from build123d import *

# Parameters (mm, degrees)
F1_DEPTH = 19.05
F2_R     = 2.5
F3_DEPTH = 1.9
F4_R     = 1.5
F5_DEPTH = 1.9


with BuildPart() as f1:
    # F0 (on Front) → F1 (new body)
    with BuildSketch(Plane.XZ):
        with BuildLine():
            Line((-18.746637599, 0), (31.253362401, 0))
            Line((31.253362401, 0), (31.253362401, 1.9))
            Line((31.253362401, 1.9), (-18.746637599, 1.9))
            ThreePointArc((-18.746637599, 1.9), (-21.0563364303, 3.4432914191), (-20.514404552, 6.167766953))
            Line((-20.514404552, 6.167766953), (-2.8367350223, 23.8454364826))
            Line((-2.8367350223, 23.8454364826), (-4.1802379066, 25.1889393669))
            Line((-4.1802379066, 25.1889393669), (-21.8579074362, 7.5112698372))
            ThreePointArc((-21.8579074362, 7.5112698372), (-22.8117075421, 2.7161928976), (-18.746637599, 0))
        make_face()
    extrude(amount=F1_DEPTH)

    # F2 (on face) → F3 (cut, through all)
    with BuildSketch(Plane.XY.offset(1.9)):
        with Locations((-0.746637599, -9.525)):
            Circle(F2_R)
        with BuildLine():
            ThreePointArc((24.1869203746, -12.025), (26.6482556642, -9.525), (24.1869203746, -7.025))
            Line((24.1869203746, -7.025), (24.1089835763, -7.025))
            Line((24.1089835763, -7.025), (14.3277980387, -7.025))
            ThreePointArc((14.3277980387, -7.025), (11.8277980387, -9.525), (14.3277980387, -12.025))
            Line((14.3277980387, -12.025), (24.1869203746, -12.025))
        make_face()
        with BuildLine():
            Line((24.1089835763, -7.025), (24.1869203746, -7.025))
            ThreePointArc((24.1869203746, -7.025), (24.1479519755, -7.0246963112), (24.1089835763, -7.025))
        make_face()
    extrude(amount=-F3_DEPTH, mode=Mode.SUBTRACT)

    # F4 (on face) → F5 (cut, through all)
    with BuildSketch(Plane(origin=(-14.6845886367, 0, 14.6845886367), x_dir=(0, -1, 0), z_dir=(-0.7071067812, 0, 0.7071067812))):
        with Locations((14.55, 7.3553952665)):
            Circle(F4_R)
        with Locations((4.5, 7.3553952665)):
            Circle(F4_R)
    extrude(amount=-F5_DEPTH, mode=Mode.SUBTRACT)


solid = f1.part
Design review of the part built by this model. Coordinates are the model's own, in mm. A direction names the side the tool comes from. Round coordinates to 2 decimals unless told otherwise and drop trailing zeros. Order: outer loops, then holes, each group sorted by start corner. A loop starts at its lowest first (then second) coordinate and runs counter-clockwise, first axis right, second up.
1) For L1, parallel to X at y = -10.25, z = 1.25; L2, parallel to X at y = -10, z = 1.25; L3, parallel to Z at x = -18.5, y = -4, list the stretches that pass through material, from the lowest coordinate up.
The answers:
L1: x = -21.82 to -3.14, 1.65 to 11.94, 26.54 to 31.25
L2: x = -21.82 to -3.2, 1.71 to 11.87, 26.6 to 31.25
L3: z = 0 to 1.9, 8.18 to 10.87
2) Consider section C-C (y = -8.75). State the section outline as (x, z) points, plus the area to 3 significant figures.
The answers:
outline: (-21.86, 7.51) arc R4.4 ccw to (-18.75, 0) - (-3.12, 0) - (-3.12, 1.9) - (-18.75, 1.9) arc R2.5 cw to (-20.51, 6.17) - (-2.84, 23.85) - (-4.18, 25.19) - close; (1.63, 0) - (11.95, 0) - (11.95, 1.9) - (1.63, 1.9) - close; (26.53, 0) - (31.25, 0) - (31.25, 1.9) - (26.53, 1.9) - close
area: 121 mm2
3) Consider section B-B (y = -15). State the section outline as (x, z) points, plus the area to 3 significant figures.
The answers:
outline: (-21.86, 7.51) arc R4.4 ccw to (-18.75, 0) - (31.25, 0) - (31.25, 1.9) - (-18.75, 1.9) arc R2.5 cw to (-20.51, 6.17) - (-9.15, 17.53) - (-10.5, 18.87) - close; (-8.47, 20.9) - (-7.13, 19.55) - (-2.84, 23.85) - (-4.18, 25.19) - close
area: 153 mm2
4) Machinability: for faces 5 (the flat face through (-11.8, -9.39, 14.88)), 6 (the flat face through (-3.5, -9.39, 24.51)), 7 (the flat face through (19, -7.025, 1)), which of the approach directions +Z, -Z, +X, -X, +Y, -Y give a long, thin tool a straight path to every point of the face, cutting with its end or side? Answer none if there is none.
The answers:
face 5: +X, +Y, -Y
face 6: +Z, +X, +Y, -Y
face 7: +Z, -Z
5) Draft analysis for pull direction Z (two halves, no side actions). For faces 1 (the cylindrical face through (-9.227, -15.936, 18.817)), 2 (the flat face through (7, -9, 1.9)), 3 (the flat face through (31.253, -9, 1)), 4 (the flat face through (6, -9, 0)), state which applies: released by +Z, released by -Z, zero draft, split by the parting line, or undercut.
The answers:
face 1: undercut
face 2: undercut
face 3: zero draft
face 4: released by -Z
6) Consider section A-A (x = 13). State the section outline as (y, z) points, plus the area to 3 significant figures.
The answers:
outline: (-19.05, 0) - (-11.64, 0) - (-11.64, 1.9) - (-19.05, 1.9) - close; (-7.41, 0) - (0, 0) - (0, 1.9) - (-7.41, 1.9) - close
area: 28.1 mm2
7) Clearance check with flat-ended pins moving along their axes: pin 1 Ø8 at (y, z) = (-4, 12.5) entering from +X; pin 2 Ø8 at (y, z) = (-9.5, 17) entering from -X; pin 3 Ø4.5 at (x, y) = (-0.75, -9.52) entering from -Z. State where each tip first meets the part, or that it passes through.
The answers:
pin 1: stops at x = -10.18
pin 2: stops at x = -16.37
pin 3: stops at z = 23.68
8) Consider section D-D (z = 2.5). State the section outline as (x, y) points, plus the area to 3 significant figures.
The answers:
outline: (-22.72, -19.05) - (-20.37, -19.05) - (-20.37, 0) - (-22.72, 0) - close
area: 44.6 mm2
